Verification items for this drawing (mm, ordinates from the low corner). A direction names the side the tool comes from. Round coordinates to 2 decimals unless told otherwise and drop trailing zeros. Loops run counter-clockwise (first coordinate to the right, second up) from the corner with the lowest first, then second, coordinate; pieces in that order, holes last. Notation, with made-up numbers: M 49.5,-3.75 L 55.5,-3.75 A25 ccw 55.5,25.25 Z; hole C 64,3.25 d1. An arc over 180 degrees is marked long. Write item = value, one per line.
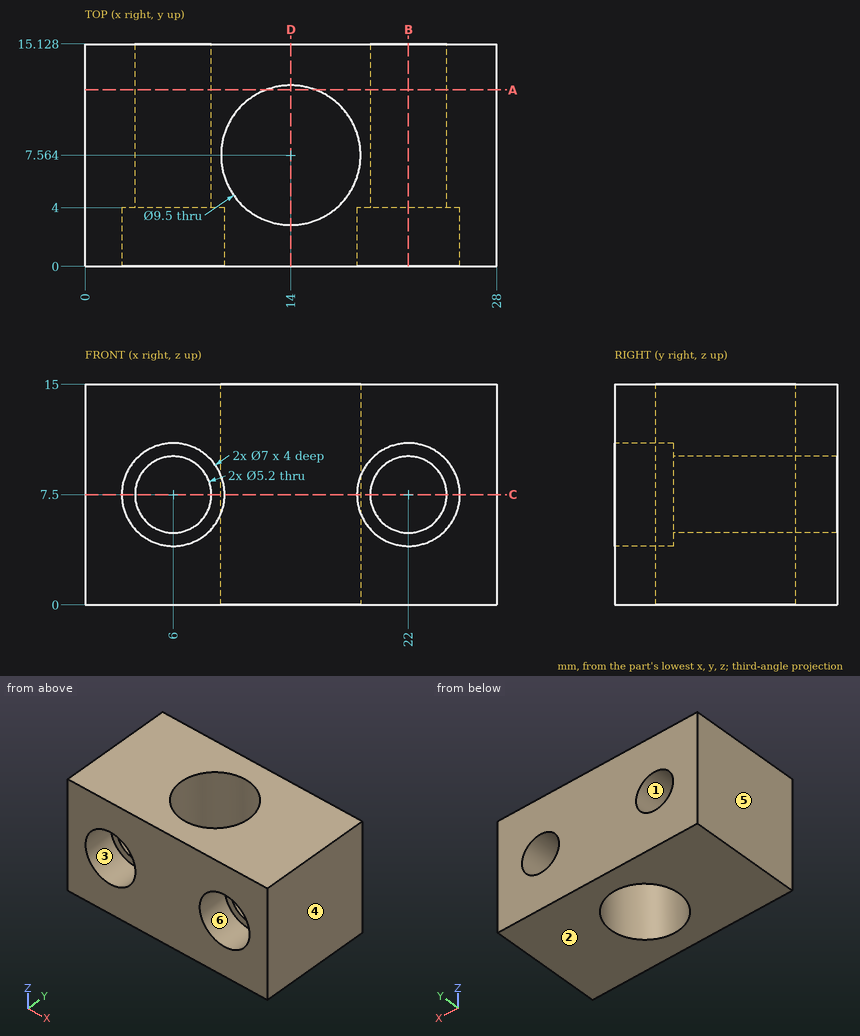
(1) Tool access check on the marked faces 5 and 6. Record the directions out of +Z, -Z, +X, -X, +Y, -Y that give a thin tool (end or side, any length) a straight path to the whole face; none if there is none.
Result set:
face_5 = +Z, -Z, -X, +Y, -Y
face_6 = -Y
(2) Sectioned sample at B-B on x = 22. Record the cut outline in (y, z), then the cut area to 3 significant figures.
Result set:
outline = M 0,0 L 15.13,0 L 15.13,4.9 L 4,4.9 L 4,4 L 0,4 Z; M 0,11 L 4,11 L 4,10.1 L 15.13,10.1 L 15.13,15 L 0,15 Z
area = 141 mm2
(3) Sectioned sample at A-A on y = 12. Record the cut outline in (x, z).
Result set:
outline = M 0,0 L 12.3,0 L 12.3,15 L 0,15 Z; M 15.7,0 L 28,0 L 28,15 L 15.7,15 Z; hole C 6,7.5 d5.2; hole C 22,7.5 d5.2
(4) Material ranges on line 1 along Z through (x, y) = (22, 2.05); line 2 along Z through (x, y) = (22, 7.5); line 3 along X through (y, z) = (5.5, 6.75), recorded low to high. Write a range as from..to.
Result set:
line_1 = 0..4, 11..15
line_2 = 0..4.9, 10.1..15
line_3 = 0..3.51, 8.49..9.72, 18.28..19.51, 24.49..28
(5) Release check for a two-part mould opening along Z. For the marked faces 1, 2, 3 and 4 record: released by +Z, released by -Z, zero draft, split by the parting line, or undercut.
Result set:
face_1 = undercut
face_2 = released by -Z
face_3 = undercut
face_4 = zero draft
(6) Sectioned sample at D-D on x = 14. Record the cut outline in (y, z).
Result set:
outline = M 0,0 L 2.81,0 L 2.81,15 L 0,15 Z; M 12.31,0 L 15.13,0 L 15.13,15 L 12.31,15 Z
(7) Sectioned sample at C-C on z = 7.5. Record the cut outline in (x, y).
Result set:
outline = M 0,0 L 2.5,0 L 2.5,4 L 3.4,4 L 3.4,15.13 L 0,15.13 Z; M 8.6,4 L 9.5,4 L 9.5,0 L 18.5,0 L 18.5,4 L 19.4,4 L 19.4,15.13 L 8.6,15.13 Z; M 24.6,4 L 25.5,4 L 25.5,0 L 28,0 L 28,15.13 L 24.6,15.13 Z; hole C 14,7.56 d9.5
(8) Depth check by flat-ended pin: pin 1 Ø5.5 at (x, y) = (14, 7.56) entering from +Z; pin 2 Ø5.5 at (x, z) = (22, 7.5) entering from -Y. Enter the tip coordinate at first touch or a pass-through.
Result set:
pin_1 = through
pin_2 = 4
